Geometry: see drawing. Coordinates: mm, zero at the bounding-box minimum. A direction names the side the tool comes from. Coordinates: 2 decimals unless noted, no trailing zeros. Loops run counter-clockwise (first coordinate to the right, second up) from the corner with the lowest first, then second, coordinate; pieces in that order, holes last. Notation, with made-up numbers: (-5.5, 8) - (27.5, 8) arc R17 ccw to (27.5, 15) - close; hole circle Ø11 at (20.25, 63). An arc over 180 degrees is marked (long way). Use one line per item in the form item = value.
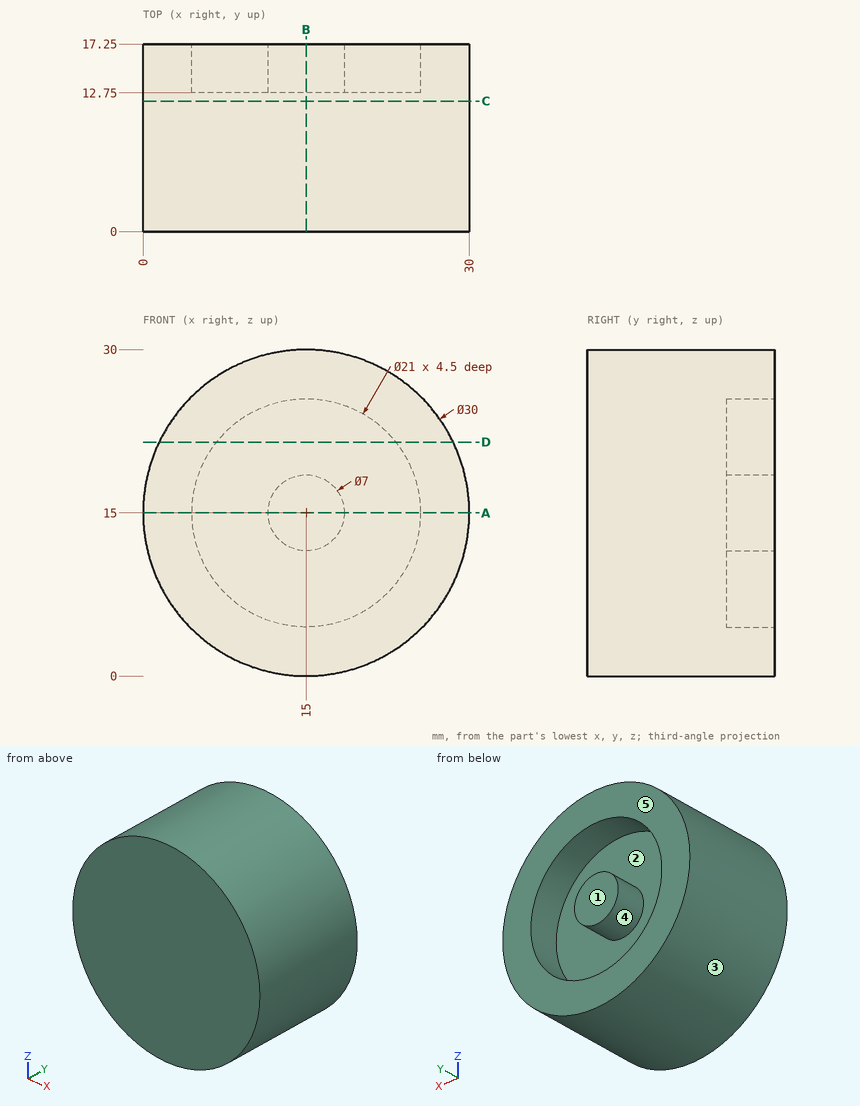
Q1. Cut plane C-C, the plane y = 12. Return loops of the section in (x, z), then the cut area to 3 significant figures.
Check values:
outline = circle Ø30 at (15, 15)
area = 707 mm²
Q2. Pull-direction query (X, two-part tool) for the marked faces 3, 4 and 5; classes: pulls with the +X half, pulls with the -X half, needs draft (parallel to the pull), parting line crosses it, or undercut.
Check values:
face_3 = parting line crosses it
face_4 = undercut
face_5 = needs draft
Q3. Cut plane B-B, the plane x = 15. Return loops of the section in (y, z), then the cut area to 4 significant figures.
Check values:
outline = (0, 0) - (17.25, 0) - (17.25, 4.5) - (12.75, 4.5) - (12.75, 11.5) - (17.25, 11.5) - (17.25, 18.5) - (12.75, 18.5) - (12.75, 25.5) - (17.25, 25.5) - (17.25, 30) - (0, 30) - close
area = 454.5 mm²
Q4. Cut plane D-D, the plane z = 21.5. Return loops of the section in (x, y).
Check values:
outline = (1.48, 0) - (28.52, 0) - (28.52, 17.25) - (23.25, 17.25) - (23.25, 12.75) - (6.75, 12.75) - (6.75, 17.25) - (1.48, 17.25) - close
Q5. Set-up query: the marked faces 1 and 2. Return all of +Z, -Z, +X, -X, +Y, -Y with unobstructed straight access to the full face (end or side cutting, diameter ignored); none if empty.
Check values:
face_1 = +Z, -Z, +X, -X, +Y
face_2 = +Y
Q6. Cut plane A-A, the plane z = 15. Return loops of the section in (x, y), then the cut area to 4 significant figures.
Check values:
outline = (0, 0) - (30, 0) - (30, 17.25) - (25.5, 17.25) - (25.5, 12.75) - (18.5, 12.75) - (18.5, 17.25) - (11.5, 17.25) - (11.5, 12.75) - (4.5, 12.75) - (4.5, 17.25) - (0, 17.25) - close
area = 454.5 mm²
Q7. First-contact query: P1, Ø6, axis at x = 18.5, y = 8.5, coming from the -Z side; P2, Ø5, axis at x = 21.5, y = 12, coming from the +Z side; P3, Ø3, axis at x = 11.5, y = 9, coming from the +Z side. Flat tips, straight axial feed; report the tip coordinate or a pass-through.
Check values:
P1 = 0.01
P2 = 29.46
P3 = 29.87
Q8. Ray query, line 1 along Z through (x, y) = (15, 14.7); line 2 along X through (y, z) = (16, 16.25); line 3 along Y through (x, z) = (17.5, 7.25). Return the intervals inside material, ascending. Write a range as [from, to].
Check values:
line_1 = [0, 4.5], [11.5, 18.5], [25.5, 30]
line_2 = [0.05, 4.57], [11.73, 18.27], [25.43, 29.95]
line_3 = [0, 12.75]
